The model under review builds one solid part; all positions refer to its coordinate system, in mm. A direction names the side the tool comes from. Round coordinates to 2 decimals unless told otherwise and drop trailing zeros. Write each loop counter-clockwise with the first axis right and the second up, starting at its lowest first coordinate (ties: lowest second). Pieces come first, ordered by that corner, then holes. Notation, with made-up numbers: (-1.75, -35.75) -> (30.25, -35.75) arc R6 ccw to (30.25, -30.75) -> close; hole circle Ø2 at (-20, 42.5). An arc over 180 degrees is marked (long way). Answer as a JSON object with one key per item and string values. Group by question number.
1) Insertion check: pin 1 Ø1 at (x, z) = (20, 13.5) entering from -Y; pin 2 Ø1.6 at (x, z) = (-1.5, -11) entering from -Y; pin 3 Ø6 at (y, z) = (-1, 5.5) entering from -X; pin 4 Ø1.9 at (x, z) = (-1.6, -10) entering from +Y. Each pin has a flat end and moves straight along its axis. Give the tip position at first contact, or say it passes through.
2) Mouldability with a two-part tool opening along Y and no side actions: class faces 6 (the flat face through (-0.206, 4.321, -7.63)), 7 (the cylindrical face through (15.65, 0.06, -16.52)), 8 (the flat face through (11, 2.8, -11)) as pulls with the +Y half, pulls with the -Y half, needs draft (parallel to the pull), parting line crosses it, or undercut.
3) Machinability: for faces 1 (the flat face through (25.9, 6, 0)), 2 (the flat face through (1.15, 4, 10)), 3 (the flat face through (8, 4.8, 0)), 4 (the cylindrical face through (15.65, 0.06, 16.52)), 5 (the flat face through (11, 2.8, 10)), which of the approach directions +Z, -Z, +X, -X, +Y, -Y give a long, thin tool a straight path to every point of the face, cutting with its end or side? Answer none if there is none.
4) We need section D-D, the plane z = 4.5. Write out the cut boundary in (x, y), then the cut area to 4 significant figures.
5) To check wall thickness, follow probe 1 along X at (y, z) = (0, -15.6); probe 2 along Z at (x, y) = (-1.6, 8.1); probe 3 along Z at (x, y) = (-4.5, 2.5). State the ranges of each line that lie inside material, in increasing order. Write a range as [from, to].
6) We need section A-A, the plane z = -10. Write out the cut boundary in (x, y), then the cut area to 3 significant figures.
7) We need section B-B, the plane y = 0. Write out the cut boundary in (x, z).
8) We need section C-C, the plane x = 22. Write out the cut boundary in (y, z), then the cut area to 3 significant figures.
from build123d import *

# Parameters (mm, degrees)
BOSS_EXTRUDE1_DEPTH        = 18
CROQUIS2_R                 = 1.35
CORTAR_EXTRUIR2_DEPTH      = 5
CORTAR_EXTRUIR3_START      = 3
CORTAR_EXTRUIR3_DEPTH      = 17
CORTAR_EXTRUIR4_DEPTH      = 33.203415968
CORTAR_EXTRUIR4_DEPTH_BACK = 2
CROQUIS4_W                 = 70
CROQUIS4_H                 = 12
CORTAR_EXTRUIR5_DEPTH      = 2.5
CORTAR_EXTRUIR5_DEPTH_BACK = 3
CROQUIS7_R                 = 0.161098749
CROQUIS7_R_2               = 1.55
CORTAR_EXTRUIR6_DEPTH      = 33.203415968


with BuildPart() as part:
    # Sketch1 → Boss-Extrude1 (new body)
    with BuildSketch(Plane.XY):
        Polygon((25.9, 9.3), (-9.1, 9.3), (-9.1, 2.5), (-9.1, -2.7), (25.9, -2.7), (25.9, 2.5), align=None)
    boss_extrude1 = extrude(amount=BOSS_EXTRUDE1_DEPTH)

    # Croquis2 → Cortar-Extruir2 (cut)
    with BuildSketch(Plane.XY.offset(18)):
        Circle(CROQUIS2_R)
        with Locations((17, 0)):
            Circle(CROQUIS2_R)
    cortar_extruir2 = extrude(amount=-CORTAR_EXTRUIR2_DEPTH, mode=Mode.SUBTRACT)

    # Croquis3 → Cortar-Extruir3 (cut)
    with BuildSketch(Plane(origin=(0, 0, 18), x_dir=(-1, 0, 0), z_dir=(0, 0, -1)).offset(CORTAR_EXTRUIR3_START)):
        Polygon((-25.9, -2.7), (-25.9, 2.8), (4.1, 2.8), (9.1, -2.2), (9.1, -2.7), align=None)
    cortar_extruir3 = extrude(amount=CORTAR_EXTRUIR3_DEPTH, mode=Mode.SUBTRACT)

    # Mirror1: Boss-Extrude1, Cortar-Extruir2, Cortar-Extruir3 across plane
    add(boss_extrude1.mirror(Plane.XY))
    add(cortar_extruir2.mirror(Plane.XY), mode=Mode.SUBTRACT)
    add(cortar_extruir3.mirror(Plane.XY), mode=Mode.SUBTRACT)

    # Croquis4 → Cortar-Extruir4 (cut, two sides: drawn at the far end of the back side and taken through both)
    with BuildSketch(Plane.XZ.offset(-2.8).offset(-CORTAR_EXTRUIR4_DEPTH_BACK)):
        with Locations((-9.1, 0)):
            Rectangle(CROQUIS4_W, CROQUIS4_H)
    extrude(amount=CORTAR_EXTRUIR4_DEPTH + CORTAR_EXTRUIR4_DEPTH_BACK, mode=Mode.SUBTRACT)

    # Croquis5 → Cortar-Extruir5 (cut, two sides: drawn at the far end of the back side and taken through both)
    with BuildSketch(Plane.XZ.offset(-2.8).offset(-CORTAR_EXTRUIR5_DEPTH_BACK)):
        Polygon((-1.6, 13.175426481), (-4.35, 11.58771324), (-4.35, 8.41228676), (-1.6, 6.824573519), (1.15, 8.41228676), (1.15, 11.58771324), align=None)
        Polygon((18.4, 13.175426481), (15.65, 11.58771324), (15.65, 8.41228676), (18.4, 6.824573519), (21.15, 8.41228676), (21.15, 11.58771324), align=None)
        Polygon((-1.6, -6.824573519), (-4.35, -8.41228676), (-4.35, -11.58771324), (-1.6, -13.175426481), (1.15, -11.58771324), (1.15, -8.41228676), align=None)
        Polygon((18.4, -6.824573519), (15.65, -8.41228676), (15.65, -11.58771324), (18.4, -13.175426481), (21.15, -11.58771324), (21.15, -8.41228676), align=None)
    extrude(amount=CORTAR_EXTRUIR5_DEPTH + CORTAR_EXTRUIR5_DEPTH_BACK, mode=Mode.SUBTRACT)

    # Croquis7 → Cortar-Extruir6 (cut, through all)
    with BuildSketch(Plane.XZ.offset(-2.8)):
        with Locations((-69.565345843, 7.024441215)):
            Circle(CROQUIS7_R)
        with Locations((-1.6, 10)):
            Circle(CROQUIS7_R_2)
        with Locations((18.4, 10)):
            Circle(CROQUIS7_R_2)
        with Locations((18.4, -10)):
            Circle(CROQUIS7_R_2)
        with Locations((-1.6, -10)):
            Circle(CROQUIS7_R_2)
    extrude(amount=-CORTAR_EXTRUIR6_DEPTH, mode=Mode.SUBTRACT)


solid = part.part
Here are the results:
{
 "1": {"pin 1": "stops at y = 2.8", "pin 2": "stops at y = 5.8", "pin 3": "stops at x = -9.1", "pin 4": "passes through"},
 "2": {"face 6": "needs draft", "face 7": "undercut", "face 8": "pulls with the -Y half"},
 "3": {"face 1": "+Z, -Z, +X, +Y, -Y", "face 2": "-Y", "face 3": "+X, -X, -Y", "face 4": "+Z, -Z", "face 5": "+X, -Y"},
 "4": {"outline": "(-9.1, 4.8) -> (25.9, 4.8) -> (25.9, 9.3) -> (-9.1, 9.3) -> close", "area": "157.5 mm^2"},
 "5": {"probe 1": "x = [-9.1, -1.35], [1.35, 15.65], [18.35, 25.9]", "probe 2": "z = [-18, -11.55], [-8.45, 8.45], [11.55, 18]", "probe 3": "z = [-18, -6], [6, 18]"},
 "6": {"outline": "(-9.1, -2.2) -> (-4.35, 2.55) -> (-4.35, 5.8) -> (-3.15, 5.8) -> (-3.15, 9.3) -> (-9.1, 9.3) -> close; (-0.05, 5.8) -> (1.15, 5.8) -> (1.15, 2.8) -> (15.65, 2.8) -> (15.65, 5.8) -> (16.85, 5.8) -> (16.85, 9.3) -> (-0.05, 9.3) -> close; (19.95, 5.8) -> (21.15, 5.8) -> (21.15, 2.8) -> (25.9, 2.8) -> (25.9, 9.3) -> (19.95, 9.3) -> close", "area": "185 mm^2"},
 "7": {"outline": "(-9.1, -18) -> (-1.35, -18) -> (-1.35, -15) -> (-6.9, -15) -> (-6.9, -6) -> (-9.1, -6) -> close; (-9.1, 6) -> (-6.9, 6) -> (-6.9, 15) -> (-1.35, 15) -> (-1.35, 18) -> (-9.1, 18) -> close; (1.35, -18) -> (15.65, -18) -> (15.65, -15) -> (1.35, -15) -> close; (1.35, 15) -> (15.65, 15) -> (15.65, 18) -> (1.35, 18) -> close; (18.35, -18) -> (25.9, -18) -> (25.9, -15) -> (18.35, -15) -> close; (18.35, 15) -> (25.9, 15) -> (25.9, 18) -> (18.35, 18) -> close"},
 "8": {"outline": "(-2.7, -18) -> (9.3, -18) -> (9.3, 18) -> (-2.7, 18) -> (-2.7, 15) -> (2.8, 15) -> (2.8, 6) -> (4.8, 6) -> (4.8, -6) -> (2.8, -6) -> (2.8, -15) -> (-2.7, -15) -> close", "area": "243 mm^2"}
}
